Input: part model. Units: mm. Frame: model coordinates. A direction names the side the tool comes from. Round coordinates to 2 decimals unless told otherwise and drop trailing zeros. Loops run counter-clockwise (first coordinate to the right, second up) from the corner with the lowest first, then second, coordinate; pieces in that order, holes last. Notation, with made-up numbers: M 11,-1 L 24,-1 A26 cw 24,21 Z; hole C 75.25,4 d9. An arc over 180 degrees is marked long. Use one line per item in the form item = value. Start each with the question number.
Q1. Section query A-A, the plane z = 6.5. Output: boundary loops of the cut face in (x, y), and give its area (3 significant figures).
Q2. First-contact query: P1, Ø9.5, axis at x = 0, y = 40, coming from the -Z side; P2, Ø2.5, axis at y = 7.5, z = 5, coming from the -X side; P3, Ø6, axis at x = 28.5, z = 6, coming from the +Y side; P4, Ø1.5, axis at x = 37.5, z = 2.5, coming from the -Y side. Flat tips, straight axial feed; report the tip coordinate or a pass-through.
Q3. Access query for faces 5 (the flat face through (1, 21, 10)), 6 (the flat face through (37, 15, 5)), 7 (the flat face through (-2, 34, 5)), 8 (the flat face through (-35, 10, 5)), 9 (the flat face through (-25, 5, 5)). Directions: +Z, -Z, +X, -X, +Y, -Y. A direction counts if a zero-diameter tool reaches every point of the face in a straight line with its end or side. Return the directions, or none.
Q4. Ray query, line 1 along X through (y, z) = (9, 6.75); line 2 along Y through (x, z) = (0, 7.25); line 3 along Y through (x, z) = (0, 3.75). Return the intervals inside material, ascending.
Q5. Section query B-B, the plane x = 0. Output: boundary loops of the cut face in (y, z), and give its area (3 significant figures).
Q6. Mould query, pull axis X, two halves, no side actions, for faces 1 (the flat face through (27, 10, 5)), 2 (the cylindrical face through (24.4, 31.9, 0.3)), 3 (the flat face through (32, 5, 5)), 4 (the cylindrical face through (0, 53, 5)). Classes: pulls with the +X half, pulls with the -X half, needs draft (parallel to the pull), parting line crosses it, or undercut.
```python
from build123d import *

# Parameters (mm, degrees)
PAD_DEPTH       = 10
SKETCH001_R     = 8
POCKET_DEPTH    = 5
SKETCH003_R     = 6
POCKET001_DEPTH = 5
POCKET002_DEPTH = 10
FILLET_R        = 1


with BuildPart() as part:
    # Sketch → Pad (new body)
    with BuildSketch(Plane.XY):
        with BuildLine():
            Line((40, 0), (-40, 0))
            Line((-40, 0), (-40, 15))
            Line((-9.661357, 48.698171), (-40, 15))
            ThreePointArc((9.661357, 48.698171), (0, 53), (-9.661357, 48.698171))
            Line((9.661357, 48.698171), (40, 15))
            Line((40, 0), (40, 15))
        make_face()
    extrude(amount=PAD_DEPTH)

    # Sketch001 → Pocket (cut)
    with BuildSketch(Plane(origin=(0, 0, 0), x_dir=(1, 0, 0), z_dir=(0, 0, -1))):
        with Locations((0, -40)):
            Circle(SKETCH001_R)
    extrude(amount=-POCKET_DEPTH, mode=Mode.SUBTRACT)

    # Sketch003 → Pocket001 (cut)
    with BuildSketch(Plane(origin=(0, 0, 5), x_dir=(1, 0, 0), z_dir=(0, 0, -1))):
        with Locations((0, -40)):
            Circle(SKETCH003_R)
    extrude(amount=-POCKET001_DEPTH, mode=Mode.SUBTRACT)

    # Sketch002 → Pocket002 (cut)
    with BuildSketch(Plane(origin=(0, 0, 0), x_dir=(1, 0, 0), z_dir=(0, 0, -1))):
        Polygon((-40, -15), (-40, 0), (-25, 0), (-25, -10), (-30, -10), (-30, -5), (-35, -5), (-35, -15), align=None)
        Polygon((40, -15), (40, 0), (25, 0), (25, -10), (30, -10), (30, -5), (35, -5), (35, -15), align=None)
    extrude(amount=-POCKET002_DEPTH, mode=Mode.SUBTRACT)

    # Fillet
    fillet_edges = [part.edges().sort_by_distance(p)[0] for p in [
        (-24.830678, 31.849086, 10),
        (-24.830678, 31.849086, 0),
    ]]
    fillet(fillet_edges, radius=FILLET_R)


solid = part.part
```
Results found:
q1.outline = M -40,15 L -35,15 L -35,5 L -30,5 L -30,10 L -25,10 L -25,0 L 25,0 L 25,10 L 30,10 L 30,5 L 35,5 L 35,15 L 40,15 L 9.66,48.7 A13 ccw -9.66,48.7 Z; hole C 0,40 d12
q1.area = 2,520 mm²
q2.P1 = through
q2.P2 = -35
q2.P3 = 31.11
q2.P4 = 15
q3.face_5 = +Z, +X, -X, +Y, -Y
q3.face_6 = +Z, -Z, +X, -Y
q3.face_7 = -Z
q3.face_8 = +Z, -Z, -X, -Y
q3.face_9 = +Z, -Z, -Y
q4.line_1 = -35 to -30, -25 to 25, 30 to 35
q4.line_2 = 0 to 34, 46 to 53
q4.line_3 = 0 to 32, 48 to 53
q5.outline = M 0,0 L 32,0 L 32,5 L 34,5 L 34,10 L 0,10 Z; M 46,5 L 48,5 L 48,0 L 52,0 A1 ccw 53,1 L 53,9 A1 ccw 52,10 L 46,10 Z
q5.area = 390 mm²
q6.face_1 = undercut
q6.face_2 = pulls with the +X half
q6.face_3 = needs draft
q6.face_4 = parting line crosses it
